Input: dimensioned drawing with shaded views. Units: mm. Origin: part minimum x, y, z. A direction names the side the tool comes from. Round coordinates to 2 decimals unless told otherwise and drop trailing zeros. Loops run counter-clockwise (first coordinate to the right, second up) from the corner with the lowest first, then second, coordinate; pieces in that order, holes last. Notation, with made-up numbers: M 16.25,-20.75 L 56.25,-20.75 A26 ccw 56.25,-6.75 Z; hole C -20,37 d2. An arc over 180 degrees is marked long. Write each question's results on one line, items separated by ' | '. Start each with the question number.
1. Contact query for flat-ended pins moving along their axis: pin 1 Ø2 at (x, y) = (25, 3.5) entering from +Z; pin 2 Ø2 at (x, z) = (9, 11) entering from -Y; pin 3 Ø6 at (x, z) = (16.5, 5.5) entering from -Y; pin 4 Ø6 at (x, z) = (4.5, 4.5) entering from -Y. Output: stop coordinate, or through.
2. Section A-A on y = 5.25. Output: boundary loops of the cut face in (x, z), and give its area (3 significant figures).
3. Draft query along X for the marked faces 1, 2, 3 and 4. Return one class per face: released by +X, released by -X, zero draft, split by the parting line, or undercut.
4. Section D-D on z = 7. Output: boundary loops of the cut face in (x, y).
5. Section C-C on y = 1. Output: boundary loops of the cut face in (x, z), and give its area (3 significant figures).
6. Set-up query: the marked faces 5, 6, 7, 8 and 9. Return all of +Z, -Z, +X, -X, +Y, -Y with unobstructed straight access to the full face (end or side cutting, diameter ignored); none if empty.
7. Section B-B on x = 5. Output: boundary loops of the cut face in (y, z), and give its area (3 significant figures).
8. Ray query, line 1 (X direction, y = 7.65, z = 7); line 2 (Z direction, x = 9, y = 2.5); line 3 (Z direction, x = 5, y = 7.7). Return the intervals inside material, ascending.
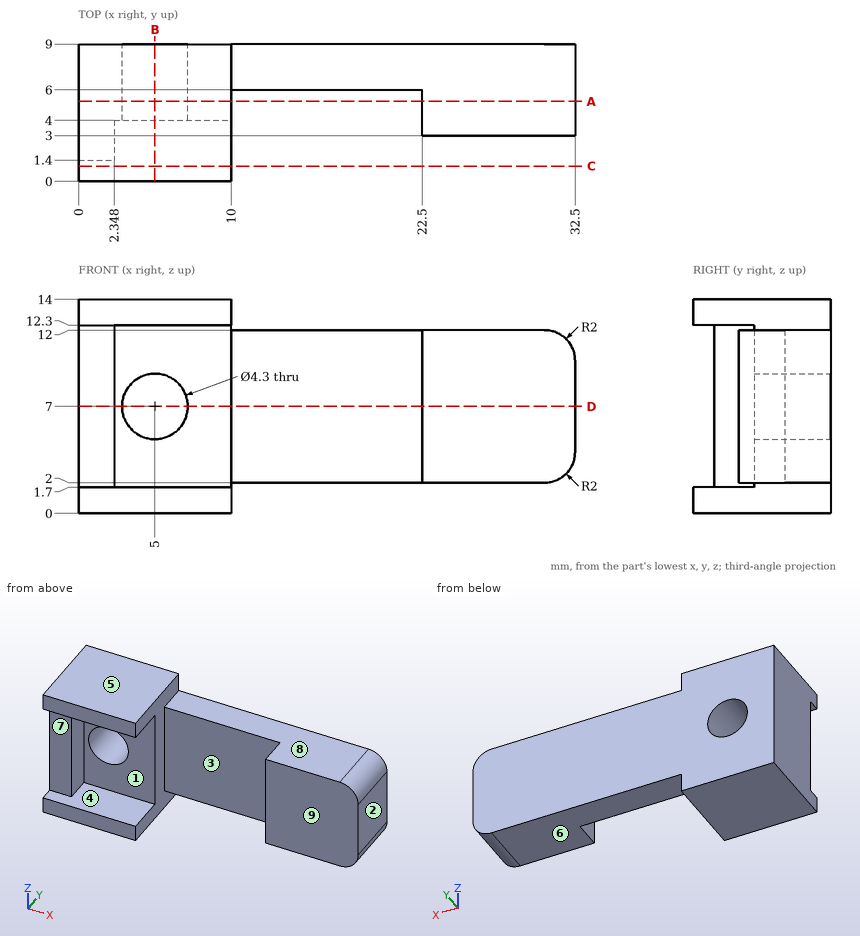
Taken from the geometry:
1) pin 1: z = 12 | pin 2: y = 4 | pin 3: y = 6 | pin 4: y = 0
2) outline: M 0,0 L 10,0 L 10,14 L 0,14 Z; M 22.5,2 L 30.5,2 A2 ccw 32.5,4 L 32.5,10 A2 ccw 30.5,12 L 22.5,12 Z; hole C 5,7 d4.3 | area: 224 mm^2
3) face 1: undercut | face 2: released by +X | face 3: undercut | face 4: zero draft
4) outline: M 0,1.4 L 2.35,1.4 L 2.35,4 L 2.85,4 L 2.85,9 L 0,9 Z; M 7.15,4 L 10,4 L 10,6 L 22.5,6 L 22.5,3 L 32.5,3 L 32.5,9 L 7.15,9 Z
5) outline: M 0,0 L 10,0 L 10,1.7 L 0,1.7 Z; M 0,12.3 L 10,12.3 L 10,14 L 0,14 Z | area: 34.0 mm^2
6) face 5: +Z, +X, -X, +Y, -Y | face 6: -Z, +X, +Y, -Y | face 7: +X, -X, -Y | face 8: +Z, +X, +Y, -Y | face 9: +Z, -Z, +X, -Y
7) outline: M 0,0 L 9,0 L 9,4.85 L 4,4.85 L 4,1.7 L 0,1.7 Z; M 0,12.3 L 4,12.3 L 4,9.15 L 9,9.15 L 9,14 L 0,14 Z | area: 62.1 mm^2
8) line 1: 0 to 2.85, 7.15 to 32.5 | line 2: 0 to 1.7, 12.3 to 14 | line 3: 0 to 4.85, 9.15 to 14
